Source: CAD feature listing. Evaluate the final solid. Frame: model axes, mm. A direction names the side the tool comes from. Give positions to 0.01 mm unless a question says otherwise; leave off trailing zeros. Write each loop counter-clockwise with the first axis right and the second up, starting at its lowest first coordinate (ties: lowest second). Pieces come first, ordered by that corner, then holes. Notation, with made-up numbers: (29, -16.5) - (45, -16.5) arc R26 ccw to (45, 20.5) - close; hole circle Ø3 at (86, 36). An arc over 180 degrees is marked (long way). Answer as a JSON object with one key per item and string values. Group by question number.
from build123d import *

# Parameters (mm, degrees)
SKETCH1_W           = 25
SKETCH1_H           = 50
SKETCH1_R           = 3.1
BOSS_EXTRUDE1_DEPTH = 3
SKETCH2_W           = 50
SKETCH2_H           = 3
BOSS_EXTRUDE2_DEPTH = 8
SKETCH3_W           = 8
SKETCH3_H           = 50
BOSS_EXTRUDE3_DEPTH = 42
SKETCH4_R           = 2.65
CUT_EXTRUDE1_DEPTH  = 3.3
SKETCH5_R           = 3.868246804
CUT_EXTRUDE2_DEPTH  = 9
FILLET2_R           = 1
SKETCH6_R           = 12.5
BOSS_EXTRUDE4_DEPTH = 2
FILLET3_R           = 1
FILLET4_R           = 1


with BuildPart() as part:
    # Sketch1 → Boss-Extrude1 (new body)
    with BuildSketch(Plane(origin=(0, 0, 0), x_dir=(1, 0, 0), z_dir=(0, 1, 0))):
        with Locations((2.276951673, 11.384758364)):
            Rectangle(SKETCH1_W, SKETCH1_H)
        with Locations(Location((1.276951673, 11.384758364, 0), (0, 0, 270))):
            Circle(SKETCH1_R, mode=Mode.SUBTRACT)
    extrude(amount=BOSS_EXTRUDE1_DEPTH)

    # Sketch2 → Boss-Extrude2 (add)
    with BuildSketch(Plane.ZY.offset(10.223048327)):
        with Locations((-11.384758364, 1.5)):
            Rectangle(SKETCH2_W, SKETCH2_H)
    extrude(amount=BOSS_EXTRUDE2_DEPTH)

    # Sketch3 → Boss-Extrude3 (add)
    with BuildSketch(Plane.XZ):
        with Locations((-14.223048327, -11.384758364)):
            Rectangle(SKETCH3_W, SKETCH3_H)
    extrude(amount=BOSS_EXTRUDE3_DEPTH)

    # Sketch4 → Cut-Extrude1 (cut)
    with BuildSketch(Plane(origin=(0, 3, 0), x_dir=(1, 0, 0), z_dir=(0, 1, 0))):
        with Locations(Location((-14.223048327, 32.384758364, 0), (0, 0, 270))):
            Circle(SKETCH4_R)
        with Locations(Location((-14.223048327, -9.615241636, 0), (0, 0, 270))):
            Circle(SKETCH4_R)
    cut_extrude1 = extrude(amount=-CUT_EXTRUDE1_DEPTH, mode=Mode.SUBTRACT)

    # Mirror1: Cut-Extrude1 across plane
    add(cut_extrude1.mirror(Plane.ZX.offset(-19.5)), mode=Mode.SUBTRACT)

    # Sketch5 → Cut-Extrude2 (cut)
    with BuildSketch(Plane.ZY.offset(18.223048327)):
        with Locations((-11.836279124, -21)):
            Circle(SKETCH5_R)
    extrude(amount=-CUT_EXTRUDE2_DEPTH, mode=Mode.SUBTRACT)

    # Fillet2
    fillet2_edges = [part.edges().sort_by_distance(p)[0] for p in [
        (-10.223048327, -21, -15.704525928),
    ]]
    fillet(fillet2_edges, radius=FILLET2_R)

    # Mirror2: Cut-Extrude1 across plane
    add(cut_extrude1.mirror(Plane.ZY.offset(1.723048327)), mode=Mode.SUBTRACT)

    # Sketch6 → Boss-Extrude4 (add)
    with BuildSketch(Plane(origin=(0, 3, 0), x_dir=(1, 0, 0), z_dir=(0, 1, 0))):
        with BuildLine():
            Line((14.776951673, 6.093255742), (14.776951673, 16.676260986))
            ThreePointArc((14.776951673, 16.676260986), (-13.223048327, 11.384758364), (14.776951673, 6.093255742))
        make_face()
        with Locations(Location((1.276951673, 11.384758364, 0), (0, 0, 270))):
            Circle(SKETCH6_R, mode=Mode.SUBTRACT)
    extrude(amount=BOSS_EXTRUDE4_DEPTH)

    # Fillet3
    fillet3_edges = [part.edges().sort_by_distance(p)[0] for p in [
        (-10.223048327, 0, -11.384758364),
    ]]
    fillet(fillet3_edges, radius=FILLET3_R)

    # Fillet4
    fillet4_edges = [part.edges().sort_by_distance(p)[0] for p in [
        (14.776951673, 5, -11.384758364),
    ]]
    fillet(fillet4_edges, radius=FILLET4_R - 0.0001)  # a hair under: the kernel refuses the full size


solid = part.part
Q1. Ray query, probe 1 along Z at (x, y) = (-15, 2); probe 2 along Y at (x, z) = (2.5, -7); probe 3 along X at (y, z) = (-36.5, 8). Return the intervals inside material, ascending. Write a range as [from, to].
Q2. Section B-B on z = -32. Return the cut outline in (x, y), then the cut area to 3 significant figures.
Q3. First-contact query: pin 1 Ø3 at (x, z) = (8, -8) entering from -Y; pin 2 Ø12.5 at (y, z) = (-17.5, -3) entering from +X; pin 3 Ø4.5 at (y, z) = (-21, -11.84) entering from -X; pin 4 Ø6 at (x, z) = (-14.22, -32.38) entering from +Y. Flat tips, straight axial feed; report the tip coordinate or a pass-through.
Q4. Section D-D on y = -14. Return the cut outline in (x, z), then the cut area to 3 significant figures.
Q5. Section A-A on y = -21. Return the cut outline in (x, z), then the cut area to 3 significant figures.
Q6. Reachability of faces 4 (the cylindrical face through (-11.596, -40.373, 9.27)), 5 (the flat face through (6, 0, -12)), 6 (the flat face through (-18.223, -14, -12)), 7 (the cylindrical face through (13.364, 1.521, -32.959)), 8 (the cylindrical face through (-9.813, 3.986, -5.617)) from +Z, -Z, +X, -X, +Y, -Y: full face, straight path, thin tool, end or side. Return the list, or none.
Q7. Draft query along Y for faces 1 (the cylindrical face through (-14.772, -24.776, -12.675)), 2 (the flat face through (-14, -42, -11)), 3 (the flat face through (-12, -14, -36.385)). Return one class per face: released by +Y, released by -Y, zero draft, split by the parting line, or undercut.
Q8. Section C-C on y = 1. Return the cut outline in (x, z).
Taken from the geometry:
{
 "1": {"probe 1": "z = [-36.38, -34.92], [-29.85, 7.08], [12.15, 13.62]", "probe 2": "y = [0, 3]", "probe 3": "x = [-18.22, -10.22]"},
 "2": {"outline": "(-18.22, -42) - (-16.84, -42) - (-16.84, -38.7) - (-11.6, -38.7) - (-11.6, -42) - (-10.22, -42) - (-10.22, -1) arc R1 cw to (-9.22, 0) - (8.16, 0) - (8.16, 3) - (-11.6, 3) - (-11.6, -0.3) - (-16.84, -0.3) - (-16.84, 3) - (-18.22, 3) - close; (13.4, 0) - (14.78, 0) - (14.78, 3) - (13.4, 3) - close", "area": "385 mm²"},
 "3": {"pin 1": "stops at y = 0", "pin 2": "stops at x = -10.22", "pin 3": "passes through", "pin 4": "stops at y = 3"},
 "4": {"outline": "(-18.22, -36.38) - (-10.22, -36.38) - (-10.22, 13.62) - (-18.22, 13.62) - close", "area": "400 mm²"},
 "5": {"outline": "(-18.22, -36.38) - (-10.22, -36.38) - (-10.22, -16.7) arc R1 ccw to (-11.22, -15.7) - (-18.22, -15.7) - close; (-18.22, -7.97) - (-11.22, -7.97) arc R1 ccw to (-10.22, -6.97) - (-10.22, 13.62) - (-18.22, 13.62) - close", "area": "338 mm²"},
 "6": {"face 4": "-Y", "face 5": "+Z, -Z, +X, -Y", "face 6": "+Z, -Z, -X, +Y, -Y", "face 7": "+Y, -Y", "face 8": "+Y"},
 "7": {"face 1": "undercut", "face 2": "released by -Y", "face 3": "zero draft"},
 "8": {"outline": "(-18.22, -36.38) - (14.78, -36.38) - (14.78, 13.62) - (-18.22, 13.62) - close; hole circle Ø5.3 at (-14.22, -32.38); hole circle Ø5.3 at (-14.22, 9.62); hole circle Ø6.2 at (1.28, -11.38); hole circle Ø5.3 at (10.78, -32.38); hole circle Ø5.3 at (10.78, 9.62)"}
}
